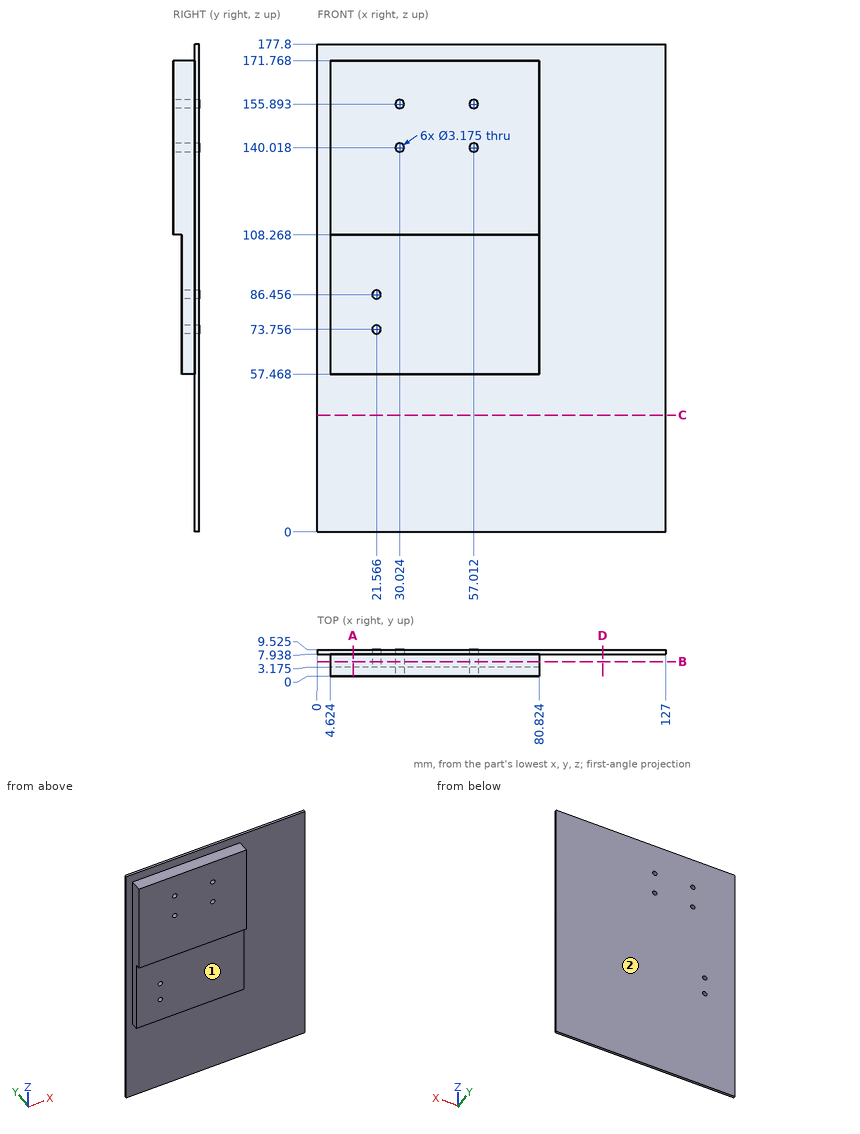
Input: dimensioned drawing with shaded views. Units: mm. Origin: part minimum x, y, z. A direction names the side the tool comes from. Coordinates: 2 decimals unless noted, no trailing zeros. Write each loop counter-clockwise with the first axis right and the second up, starting at its lowest first coordinate (ties: lowest second). Pieces come first, ordered by that corner, then holes. Notation, with made-up numbers: M 80,19.5 L 101,19.5 A29 ccw 101,55.5 Z; hole C 22.25,-2.75 d9. An arc over 180 degrees is marked long. Answer as CSV lines item,"result". Start each with the question number.
Q1. Cut plane A-A on x = 13. Return the cut outline in (y, z) (1 decimal).
Q2. Cut plane D-D on x = 104. Return the cut outline in (y, z) (1 decimal).
Q3. Reachability of the marked faces 1 and 2 from +Z, -Z, +X, -X, +Y, -Y: full face, straight path, thin tool, end or side. Return the list, or none.
Q4. Pin query (flat end, axial travel): P1, Ø3.5, axis at x = 57.01, z = 155.89, coming from the +Y side (1 decimal); P2, Ø2.5, axis at x = 21.57, z = 73.76, coming from the -Y side; P3, Ø1, axis at x = 78.5, y = 4.5, coming from the +Z side; P4, Ø2.5, axis at x = 53, y = 4.5, coming from the -Z side. Return the tip coordinate at first contact, or that it passes through.
Q5. Line query: line 1 (Z direction, x = 30, y = 4.75) (1 decimal); line 2 (X direction, y = 1, z = 163.5) (1 decimal); line 3 (Z direction, x = 59, y = 5.75). Output: solid intervals per line, ascending. Write a range as from..to.
Q6. Cut plane C-C on z = 42.5. Return the cut outline in (x, y) (1 decimal).
Q7. Cut plane B-B on y = 5.25. Return the cut outline in (x, z) (1 decimal).
Findings below:
1,outline,"M 0,108.3 L 3.2,108.3 L 3.2,57.5 L 7.9,57.5 L 7.9,0 L 9.5,0 L 9.5,177.8 L 7.9,177.8 L 7.9,171.8 L 0,171.8 Z"
2,outline,"M 7.9,0 L 9.5,0 L 9.5,177.8 L 7.9,177.8 Z"
3,face 1,"-Z, +X, -X, -Y"
3,face 2,"+Z, -Z, +X, -X, +Y"
4,P1,"stops at y = 9.5"
4,P2,"passes through"
4,P3,"stops at z = 171.77"
4,P4,"stops at z = 57.47"
5,line 1,"z = 57.5..138.4, 141.6..154.3, 157.5..171.8"
5,line 2,"x = 4.6..80.8"
5,line 3,"z = 57.47..171.77"
6,outline,"M 0,7.9 L 127,7.9 L 127,9.5 L 0,9.5 Z"
7,outline,"M 4.6,57.5 L 80.8,57.5 L 80.8,171.8 L 4.6,171.8 Z; hole C 21.6,73.8 d3.2; hole C 21.6,86.5 d3.2; hole C 30,140 d3.2; hole C 30,155.9 d3.2; hole C 57,140 d3.2; hole C 57,155.9 d3.2"
